Geometry: final body of the model. Coordinates: model frame, mm. A direction names the side the tool comes from. Give positions to 0.01 mm unless a question says otherwise; leave off trailing zeros. Write each loop counter-clockwise with the first axis right and the second up, starting at its lowest first coordinate (ties: lowest second). Pieces come first, ordered by that corner, then holes. Notation, with made-up numbers: M 62.25,30 L 117.25,30 A24 cw 117.25,54 Z; hole C 7.25,63 d2. An arc over 180 degrees is marked long. One line per question, with ' | ' between items.
from build123d import *

# Parameters (mm, degrees)
F0_W      = 139.7
F0_H      = 381
F1_DEPTH  = 2.54
F2_W      = 139.7
F2_H      = 254
F3_DEPTH  = 2.54
F4_W      = 381
F4_H      = 254
F5_DEPTH  = 2.54
F7_W      = 139.7
F7_H      = 254
F8_DEPTH  = 2.54
F10_W     = 139.7
F10_H     = 381
F11_DEPTH = 2.54
F12_W     = 5.08
F12_H     = 70.451392
F13_DEPTH = 2.54
F14_W     = 33.02
F14_H     = 33.02
F15_DEPTH = 7.62
F18_DEPTH = 2.54
F19_R     = 3.175
F20_DEPTH = 0.254
F22_DEPTH = 2.54
F24_DEPTH = 3.048
F25_W     = 38.1
F25_H     = 138.263544
F26_DEPTH = 2.54
F27_W     = 36.467261
F27_H     = 34.500528
F28_DEPTH = 43.942
F30_DEPTH = 12.954
F31_W     = 0.868231
F31_H     = 1.430023
F31_W_2   = 0.817157
F31_H_2   = 1.021446
F31_W_3   = 0.817158
F32_DEPTH = 12.446


with BuildPart() as f1:
    # F0 (on Top) → F1 (new body)
    with BuildSketch(Plane.XY):
        with Locations((69.85, 190.5)):
            Rectangle(F0_W, F0_H)
    extrude(amount=F1_DEPTH)

    # F2 (on Front) → F3 (join)
    with BuildSketch(Plane.XZ):
        with Locations((69.85, 127)):
            Rectangle(F2_W, F2_H)
    extrude(amount=F3_DEPTH)

    # F4 (on Right) → F5 (join)
    with BuildSketch(Plane.YZ):
        with Locations((190.5, 127)):
            Rectangle(F4_W, F4_H)
    extrude(amount=F5_DEPTH)

    # F7 (on offset) → F8 (join)
    with BuildSketch(Plane.XZ.offset(-381)):
        with Locations((69.85, 127)):
            Rectangle(F7_W, F7_H)
    extrude(amount=F8_DEPTH)

    # F10 (on offset) → F11 (join)
    with BuildSketch(Plane.XY.offset(254)):
        with Locations((69.85, 190.5)):
            Rectangle(F10_W, F10_H)
    extrude(amount=-F11_DEPTH)

    # F12 (on face) → F13 (cut)
    with BuildSketch(Plane.XZ.offset(2.54)):
        with Locations((40.64, 211.154304)):
            Rectangle(F12_W, F12_H)
        with Locations((30.48, 211.154304)):
            Rectangle(F12_W, F12_H)
        with Locations((20.32, 211.154304)):
            Rectangle(F12_W, F12_H)
        with Locations((10.16, 211.154304)):
            Rectangle(F12_W, F12_H)
    extrude(amount=-F13_DEPTH, mode=Mode.SUBTRACT)

    # F14 (on Front) → F15 (join)
    with BuildSketch(Plane.XZ):
        with Locations((25.453158, 213.36)):
            Rectangle(F14_W, F14_H)
        Polygon((10.213158, 228.6), (40.687077, 228.6), (40.687077, 198.12), (25.453158, 198.12), (10.213158, 198.12), align=None, mode=Mode.SUBTRACT)
    extrude(amount=-F15_DEPTH)

    # F17 (on offset) → F18 (cut)
    with BuildSketch(Plane.YZ.offset(139.7)):
        with BuildLine():
            Line((181.61, 234.763073), (181.61, 247.482779))
            ThreePointArc((181.61, 247.482779), (102.647567, 212.312433), (67.477221, 133.35))
            Line((67.477221, 133.35), (80.196927, 133.35))
            ThreePointArc((80.196927, 133.35), (111.627823, 203.332177), (181.61, 234.763073))
        make_face()
        with BuildLine():
            Line((181.61, 209.305407), (181.61, 222.038098))
            ThreePointArc((181.61, 222.038098), (120.608079, 194.351921), (92.921902, 133.35))
            Line((92.921902, 133.35), (105.654593, 133.35))
            ThreePointArc((105.654593, 133.35), (129.588335, 185.371665), (181.61, 209.305407))
        make_face()
        with BuildLine():
            Line((181.61, 183.796127), (181.61, 196.560765))
            ThreePointArc((181.61, 196.560765), (138.568591, 176.391409), (118.399235, 133.35))
            Line((118.399235, 133.35), (131.163873, 133.35))
            ThreePointArc((131.163873, 133.35), (147.548847, 167.411153), (181.61, 183.796127))
        make_face()
        with BuildLine():
            Line((181.61, 158.10852), (181.61, 170.994091))
            ThreePointArc((181.61, 170.994091), (156.529104, 158.430896), (143.965909, 133.35))
            Line((143.965909, 133.35), (156.85148, 133.35))
            ThreePointArc((156.85148, 133.35), (165.50936, 149.45064), (181.61, 158.10852))
        make_face()
        with BuildLine():
            Line((181.61, 133.35), (181.61, 144.960512))
            ThreePointArc((181.61, 144.960512), (174.489616, 140.470384), (169.999488, 133.35))
            Line((169.999488, 133.35), (181.61, 133.35))
        make_face()
        with BuildLine():
            Line((194.31, 133.35), (205.920512, 133.35))
            ThreePointArc((205.920512, 133.35), (201.430384, 140.470384), (194.31, 144.960512))
            Line((194.31, 144.960512), (194.31, 133.35))
        make_face()
        with BuildLine():
            Line((219.06852, 133.35), (231.954091, 133.35))
            ThreePointArc((231.954091, 133.35), (219.390896, 158.430896), (194.31, 170.994091))
            Line((194.31, 170.994091), (194.31, 158.10852))
            ThreePointArc((194.31, 158.10852), (210.41064, 149.45064), (219.06852, 133.35))
        make_face()
        with BuildLine():
            Line((244.756127, 133.35), (257.520765, 133.35))
            ThreePointArc((257.520765, 133.35), (237.351409, 176.391409), (194.31, 196.560765))
            Line((194.31, 196.560765), (194.31, 183.796127))
            ThreePointArc((194.31, 183.796127), (228.371153, 167.411153), (244.756127, 133.35))
        make_face()
        with BuildLine():
            Line((270.265407, 133.35), (282.998098, 133.35))
            ThreePointArc((282.998098, 133.35), (255.311921, 194.351921), (194.31, 222.038098))
            Line((194.31, 222.038098), (194.31, 209.305407))
            ThreePointArc((194.31, 209.305407), (246.331665, 185.371665), (270.265407, 133.35))
        make_face()
        with BuildLine():
            Line((295.723073, 133.35), (308.442779, 133.35))
            ThreePointArc((308.442779, 133.35), (273.272433, 212.312433), (194.31, 247.482779))
            Line((194.31, 247.482779), (194.31, 234.763073))
            ThreePointArc((194.31, 234.763073), (264.292177, 203.332177), (295.723073, 133.35))
        make_face()
        with BuildLine():
            ThreePointArc((194.31, 6.517221), (273.272433, 41.687567), (308.442779, 120.65))
            Line((308.442779, 120.65), (295.723073, 120.65))
            ThreePointArc((295.723073, 120.65), (264.292177, 50.667823), (194.31, 19.236927))
            Line((194.31, 19.236927), (194.31, 6.517221))
        make_face()
        with BuildLine():
            ThreePointArc((194.31, 31.961902), (255.311921, 59.648079), (282.998098, 120.65))
            Line((282.998098, 120.65), (270.265407, 120.65))
            ThreePointArc((270.265407, 120.65), (246.331665, 68.628335), (194.31, 44.694593))
            Line((194.31, 44.694593), (194.31, 31.961902))
        make_face()
        with BuildLine():
            ThreePointArc((194.31, 57.439235), (237.351409, 77.608591), (257.520765, 120.65))
            Line((257.520765, 120.65), (244.756127, 120.65))
            ThreePointArc((244.756127, 120.65), (228.371153, 86.588847), (194.31, 70.203873))
            Line((194.31, 70.203873), (194.31, 57.439235))
        make_face()
        with BuildLine():
            ThreePointArc((194.31, 83.005909), (219.390896, 95.569104), (231.954091, 120.65))
            Line((231.954091, 120.65), (219.06852, 120.65))
            ThreePointArc((219.06852, 120.65), (210.41064, 104.54936), (194.31, 95.89148))
            Line((194.31, 95.89148), (194.31, 83.005909))
        make_face()
        with BuildLine():
            ThreePointArc((194.31, 109.039488), (201.430384, 113.529616), (205.920512, 120.65))
            Line((205.920512, 120.65), (194.31, 120.65))
            Line((194.31, 120.65), (194.31, 109.039488))
        make_face()
        with BuildLine():
            ThreePointArc((67.477221, 120.65), (102.647567, 41.687567), (181.61, 6.517221))
            Line((181.61, 6.517221), (181.61, 19.236927))
            ThreePointArc((181.61, 19.236927), (111.627823, 50.667823), (80.196927, 120.65))
            Line((80.196927, 120.65), (67.477221, 120.65))
        make_face()
        with BuildLine():
            ThreePointArc((92.921902, 120.65), (120.608079, 59.648079), (181.61, 31.961902))
            Line((181.61, 31.961902), (181.61, 44.694593))
            ThreePointArc((181.61, 44.694593), (129.588335, 68.628335), (105.654593, 120.65))
            Line((105.654593, 120.65), (92.921902, 120.65))
        make_face()
        with BuildLine():
            ThreePointArc((118.399235, 120.65), (138.568591, 77.608591), (181.61, 57.439235))
            Line((181.61, 57.439235), (181.61, 70.203873))
            ThreePointArc((181.61, 70.203873), (147.548847, 86.588847), (131.163873, 120.65))
            Line((131.163873, 120.65), (118.399235, 120.65))
        make_face()
        with BuildLine():
            ThreePointArc((143.965909, 120.65), (156.529104, 95.569104), (181.61, 83.005909))
            Line((181.61, 83.005909), (181.61, 95.89148))
            ThreePointArc((181.61, 95.89148), (165.50936, 104.54936), (156.85148, 120.65))
            Line((156.85148, 120.65), (143.965909, 120.65))
        make_face()
        with BuildLine():
            ThreePointArc((169.999488, 120.65), (174.489616, 113.529616), (181.61, 109.039488))
            Line((181.61, 109.039488), (181.61, 120.65))
            Line((181.61, 120.65), (169.999488, 120.65))
        make_face()
    extrude(amount=-F18_DEPTH, mode=Mode.SUBTRACT)

    # F19 (on face) → F20 (join)
    with BuildSketch(Plane(origin=(0, 381, 0), x_dir=(-1, 0, 0), z_dir=(0, 1, 0))):
        with Locations((-66.46537, 234.394625)):
            Circle(F19_R)
    extrude(amount=F20_DEPTH)

    # F21 (on face) → F22 (cut)
    with BuildSketch(Plane.XZ.offset(2.54)):
        Polygon((95.25, 19.05), (95.25, 12.7), (98.90151, 10.5918), (109.37849, 10.5918), (113.03, 12.7), (113.03, 19.05), align=None)
    extrude(amount=-F22_DEPTH, mode=Mode.SUBTRACT)

    # F23 (on face) → F24 (join)
    with BuildSketch(Plane(origin=(0, 0, 0), x_dir=(1, 0, 0), z_dir=(0, 0, -1))):
        with BuildLine():
            ThreePointArc((22.86, -365.76), (9.851846, -360.371846), (15.24, -373.38))
            ThreePointArc((15.24, -373.38), (20.628154, -371.148154), (22.86, -365.76))
        make_face()
        with BuildLine():
            ThreePointArc((132.08, -365.76), (119.071846, -360.371846), (124.46, -373.38))
            ThreePointArc((124.46, -373.38), (129.848154, -371.148154), (132.08, -365.76))
        make_face()
        with BuildLine():
            ThreePointArc((132.08, -12.7), (129.848154, -7.311846), (124.46, -5.08))
            ThreePointArc((124.46, -5.08), (119.071846, -18.088154), (132.08, -12.7))
        make_face()
        with BuildLine():
            ThreePointArc((22.86, -12.7), (20.628154, -7.311846), (15.24, -5.08))
            ThreePointArc((15.24, -5.08), (9.851846, -18.088154), (22.86, -12.7))
        make_face()
    extrude(amount=F24_DEPTH)

    # F25 (on face) → F26 (cut)
    with BuildSketch(Plane.XZ.offset(2.54)):
        with Locations((22.86, 82.675149)):
            Rectangle(F25_W, F25_H)
    extrude(amount=-F26_DEPTH, mode=Mode.SUBTRACT)

    # F27 (on Front) → F28 (join)
    with BuildSketch(Plane.XZ):
        with Locations((103.505354, 19.790264)):
            Rectangle(F27_W, F27_H)
    extrude(amount=-F28_DEPTH)

    # F29 (on face) → F30 (cut)
    with BuildSketch(Plane.XZ):
        Polygon((113.03, 12.7), (113.03, 19.05), (95.25, 19.05), (95.25, 12.7), (98.90151, 10.5918), (109.37849, 10.5918), align=None)
    extrude(amount=-F30_DEPTH, mode=Mode.SUBTRACT)

    # F31 (on face) → F32 (join)
    with BuildSketch(Plane.XZ.offset(-12.954)):
        with Locations((107.827298, 16.047901)):
            Rectangle(F31_W, F31_H)
        with Locations((104.328845, 13.136782)):
            Rectangle(F31_W_2, F31_H_2)
        with Locations((100.447353, 16.047901)):
            Rectangle(F31_W_3, F31_H)
    extrude(amount=F32_DEPTH)


solid = f1.part
(1) Cut plane A-A, the plane z = 67.5. Return loops of the section in (x, y).
Working result:
outline: M 0,-2.54 L 3.81,-2.54 L 3.81,0 L 2.54,0 L 2.54,378.46 L 139.7,378.46 L 139.7,381 L 0,381 Z; M 41.91,-2.54 L 139.7,-2.54 L 139.7,0 L 41.91,0 Z
(2) Cut plane D-D, the plane y = 98. Return loops of the section in (x, z), then the cut area to 3 significant figures.
Working result:
outline: M 0,0 L 139.7,0 L 139.7,2.54 L 2.54,2.54 L 2.54,251.46 L 139.7,251.46 L 139.7,254 L 0,254 Z | area: 1,340 mm^2
(3) Cut plane B-B, the plane z = 206. Count the separate pieces of the cut face and the enclosed holes in it, then the cut area to 3 significant figures.
Working result:
separate pieces: 7 | enclosed holes: 0 | area: 1,640 mm^2
(4) Material intervals for L1, parallel to Y at x = 95.5, z = 175.5; L2, parallel to Z at x = 65.5, y = 171; L3, parallel to Y at x = 116, z = 16, sorted ascending. Write a range as [from, to].
Working result:
L1: y = [-2.54, 0], [378.46, 381] | L2: z = [0, 2.54], [251.46, 254] | L3: y = [-2.54, 43.94], [378.46, 381]
(5) Set-up query: faces 1 (the face through (25, 4, 196.85)), 2 (the face through (10.213, 4, 213)), 3 (the face through (25, 4, 228.6)). Return all of +Z, -Z, +X, -X, +Y, -Y with unobstructed straight access to the full face (end or side cutting, diameter ignored); none if empty.
Working result:
face 1: +X | face 2: -Y | face 3: none
(6) First-contact query: P1, Ø1, axis at x = 52, z = 84, coming from the +Y side; P2, Ø1, axis at x = 20, z = 197.5, coming from the -Y side; P3, Ø2, axis at x = 90, y = 242, coming from the -Z side. Flat tips, straight axial feed; report the tip coordinate or a pass-through.
Working result:
P1: stops at y = 381 | P2: stops at y = 0 | P3: stops at z = 0
(7) Cut plane C-C, the plane x = 76. Return loops of the section in (y, z), then the cut area to 3 significant figures.
Working result:
outline: M -2.54,0 L 381,0 L 381,254 L -2.54,254 Z; hole M 0,2.54 L 378.46,2.54 L 378.46,251.46 L 0,251.46 Z | area: 3,210 mm^2
(8) Draft query along Z for faces 4 (the face through (84, -2.54, 129)), 5 (the face through (70, 192, 251.46)), 6 (the face through (15, 13, -3.048)). Return one class per face: released by +Z, released by -Z, zero draft, split by the parting line, or undercut.
Working result:
face 4: zero draft | face 5: undercut | face 6: released by -Z
